The model under review builds one solid part; all positions refer to its coordinate system, in mm. A direction names the side the tool comes from. Round coordinates to 2 decimals unless told otherwise and drop trailing zeros. Loops run counter-clockwise (first coordinate to the right, second up) from the corner with the lowest first, then second, coordinate; pieces in that order, holes last. Notation, with made-up numbers: (75.5, 84.25) - (107.5, 84.25) arc R20 ccw to (107.5, 123.25) - close; hole circle Ø3 at (26, -0.5). An arc over 180 degrees is marked (long way). Answer as CSV lines item,"result".
from build123d import *

# Parameters (mm, degrees)
SKETCH1_W           = 47.498
SKETCH1_H           = 38.1
BOSS_EXTRUDE1_DEPTH = 63.5
SKETCH3_W           = 47.498
SKETCH3_H           = 10.16
CUT_EXTRUDE1_DEPTH  = 38.1
SKETCH4_W           = 41.91
SKETCH4_H           = 17.145
CUT_EXTRUDE2_DEPTH  = 19.05
SKETCH5_W           = 40.132
SKETCH5_H           = 10.16
CUT_EXTRUDE3_DEPTH  = 49.770149692
SKETCH6_W           = 9.652
SKETCH6_H           = 38.1
SKETCH6_W_2         = 4.699
CUT_EXTRUDE4_DEPTH  = 31.75


with BuildPart() as part:
    # Sketch1 → Boss-Extrude1 (new body)
    with BuildSketch(Plane(origin=(0, 0, 0), x_dir=(1, 0, 0), z_dir=(0, 1, 0))):
        Rectangle(SKETCH1_W, SKETCH1_H)
    extrude(amount=BOSS_EXTRUDE1_DEPTH)

    # Sketch3 → Cut-Extrude1 (cut)
    with BuildSketch(Plane(origin=(0, 63.5, 0), x_dir=(1, 0, 0), z_dir=(0, 1, 0))):
        Rectangle(SKETCH3_W, SKETCH3_H)
    extrude(amount=-CUT_EXTRUDE1_DEPTH, mode=Mode.SUBTRACT)

    # Sketch4 → Cut-Extrude2 (cut)
    with BuildSketch(Plane.XZ):
        with Locations((-2.794, 0)):
            Rectangle(SKETCH4_W, SKETCH4_H)
    extrude(amount=-CUT_EXTRUDE2_DEPTH, mode=Mode.SUBTRACT)

    # Sketch5 → Cut-Extrude3 (cut, through all)
    with BuildSketch(Plane(origin=(0, 25.4, 0), x_dir=(1, 0, 0), z_dir=(0, 1, 0))):
        with Locations((-1.905, 0)):
            Rectangle(SKETCH5_W, SKETCH5_H)
    extrude(amount=-CUT_EXTRUDE3_DEPTH, mode=Mode.SUBTRACT)

    # Sketch6 → Cut-Extrude4 (cut)
    with BuildSketch(Plane(origin=(0, 63.5, 0), x_dir=(1, 0, 0), z_dir=(0, 1, 0))):
        with Locations((11.684, 0)):
            Rectangle(SKETCH6_W, SKETCH6_H)
        with Locations((-21.3995, 0)):
            Rectangle(SKETCH6_W_2, SKETCH6_H)
    extrude(amount=-CUT_EXTRUDE4_DEPTH, mode=Mode.SUBTRACT)


solid = part.part
1. Take a section at D-D (z = -13). State the section outline as (x, y) points, plus the area to 3 significant figures.
Numbers:
outline,"(-23.75, 0) - (23.75, 0) - (23.75, 63.5) - (16.51, 63.5) - (16.51, 31.75) - (6.86, 31.75) - (6.86, 63.5) - (-19.05, 63.5) - (-19.05, 31.75) - (-23.75, 31.75) - close"
area,"2,560 mm²"
2. Wall thickness on probe 1 along X at (y, z) = (43.5, -8.5); probe 2 along Z at (x, y) = (2.5, 48.5); probe 3 along Z at (x, y) = (-18.5, 17.5): over which ranges is each line inside the solid? List them lowest first.
Numbers:
probe 1,"x = -19.05 to 6.86, 16.51 to 23.75"
probe 2,"z = -19.05 to -5.08, 5.08 to 19.05"
probe 3,"z = -19.05 to -8.57, 8.57 to 19.05"
3. Draft analysis for pull direction X (two halves, no side actions). For faces 1 (the face through (18.161, 13, 0)), 2 (the face through (-23, 25.4, 0)), 3 (the face through (23.749, 24, 0)), state which applies: +X half, -X half, draft (parallel to the pull), parting line (faces both ways), or undercut.
Numbers:
face 1,"undercut"
face 2,"draft"
face 3,"+X half"
4. Tool access review of faces 4 (the face through (-19.05, 48, 12)), 5 (the face through (12, 31.75, 12)), 6 (the face through (-3, 9, 8.572)): name each direction out of +Z, -Z, +X, -X, +Y, -Y from which nothing blocks a thin tool from reaching the whole face with its end or side.
Numbers:
face 4,"+Z, -Z, -X, +Y"
face 5,"+Z, -Z, +Y"
face 6,"-X, -Y"
5. Take a section at B-B (x = 11). State the section outline as (y, z) points, plus the area to 3 significant figures.
Numbers:
outline,"(0, -19.05) - (31.75, -19.05) - (31.75, -5.08) - (19.05, -5.08) - (19.05, -8.57) - (0, -8.57) - close; (0, 8.57) - (19.05, 8.57) - (19.05, 5.08) - (31.75, 5.08) - (31.75, 19.05) - (0, 19.05) - close"
area,"754 mm²"
6. Take a section at A-A (y = 29). State the section outline as (x, z) points.
Numbers:
outline,"(-23.75, -19.05) - (23.75, -19.05) - (23.75, -5.08) - (-23.75, -5.08) - close; (-23.75, 5.08) - (23.75, 5.08) - (23.75, 19.05) - (-23.75, 19.05) - close"
7. Clearance check with flat-ended pins moving along their axes: pin 1 (11 mm diameter, centred on y = 53.5, z = 15.5, fed in from -X); pin 2 (4 mm diameter, centred on x = -1.5, z = -5.5, fed in from -Y); pin 3 (1.7 mm diameter, centred on x = 22, z = -2, fed in from +Y). State where each tip first meets the part, or that it passes through.
Numbers:
pin 1,"stops at x = -19.05"
pin 2,"stops at y = 19.05"
pin 3,"stops at y = 25.4"
8. Take a section at C-C (y = 46). State the section outline as (x, z) points, plus the area to 3 significant figures.
Numbers:
outline,"(-19.05, -19.05) - (6.86, -19.05) - (6.86, -5.08) - (-19.05, -5.08) - close; (-19.05, 5.08) - (6.86, 5.08) - (6.86, 19.05) - (-19.05, 19.05) - close; (16.51, -19.05) - (23.75, -19.05) - (23.75, -5.08) - (16.51, -5.08) - close; (16.51, 5.08) - (23.75, 5.08) - (23.75, 19.05) - (16.51, 19.05) - close"
area,"926 mm²"
